Drawing for the job (mm, zero at the part's lowest x, y, z). Coordinates: 2 decimals unless noted, no trailing zeros. Order: outer loops, then holes, each group sorted by start corner. A loop starts at its lowest first (then second) coordinate and runs counter-clockwise, first axis right, second up.
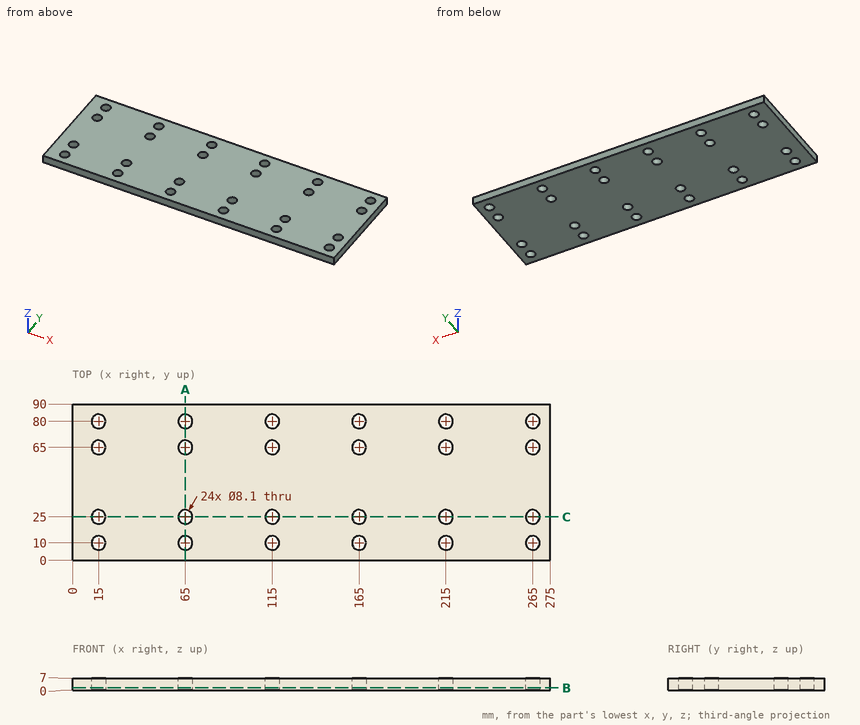
(1) Slice it at A-A, the plane x = 65. Give the cut face in (y, z), then the cut area to 3 significant figures.
(2) Slice it at C-C, the plane y = 25. Give the cut face in (x, z), then the cut area to 3 significant figures.
(3) Slice it at B-B, the plane z = 1.5. State how many separate pieces and enclosed holes the cut face has, then the cut area to 3 significant figures.
(4) Probe line 1 (Y direction, x = 165, z = 3.75); line 2 (Y direction, x = 16, z = 6). List the from-to ranges inside material, lowest first.
(5) Drop a flat-ended pin along its axis: pin 1 (5 mm diameter, centred on x = 215, y = 80, fed in from -Z). Give the stop position or say it passes through.
Here are the results:
1. outline: (0, 0) - (5.95, 0) - (5.95, 7) - (0, 7) - close; (14.05, 0) - (20.95, 0) - (20.95, 7) - (14.05, 7) - close; (29.05, 0) - (60.95, 0) - (60.95, 7) - (29.05, 7) - close; (69.05, 0) - (75.95, 0) - (75.95, 7) - (69.05, 7) - close; (84.05, 0) - (90, 0) - (90, 7) - (84.05, 7) - close
1. area: 403 mm2
2. outline: (0, 0) - (10.95, 0) - (10.95, 7) - (0, 7) - close; (19.05, 0) - (60.95, 0) - (60.95, 7) - (19.05, 7) - close; (69.05, 0) - (110.95, 0) - (110.95, 7) - (69.05, 7) - close; (119.05, 0) - (160.95, 0) - (160.95, 7) - (119.05, 7) - close; (169.05, 0) - (210.95, 0) - (210.95, 7) - (169.05, 7) - close; (219.05, 0) - (260.95, 0) - (260.95, 7) - (219.05, 7) - close; (269.05, 0) - (275, 0) - (275, 7) - (269.05, 7) - close
2. area: 1,580 mm2
3. separate pieces: 1
3. enclosed holes: 24
3. area: 23,500 mm2
4. line 1: y = 0 to 5.95, 14.05 to 20.95, 29.05 to 60.95, 69.05 to 75.95, 84.05 to 90
4. line 2: y = 0 to 6.08, 13.92 to 21.08, 28.92 to 61.08, 68.92 to 76.08, 83.92 to 90
5. pin 1: passes through
